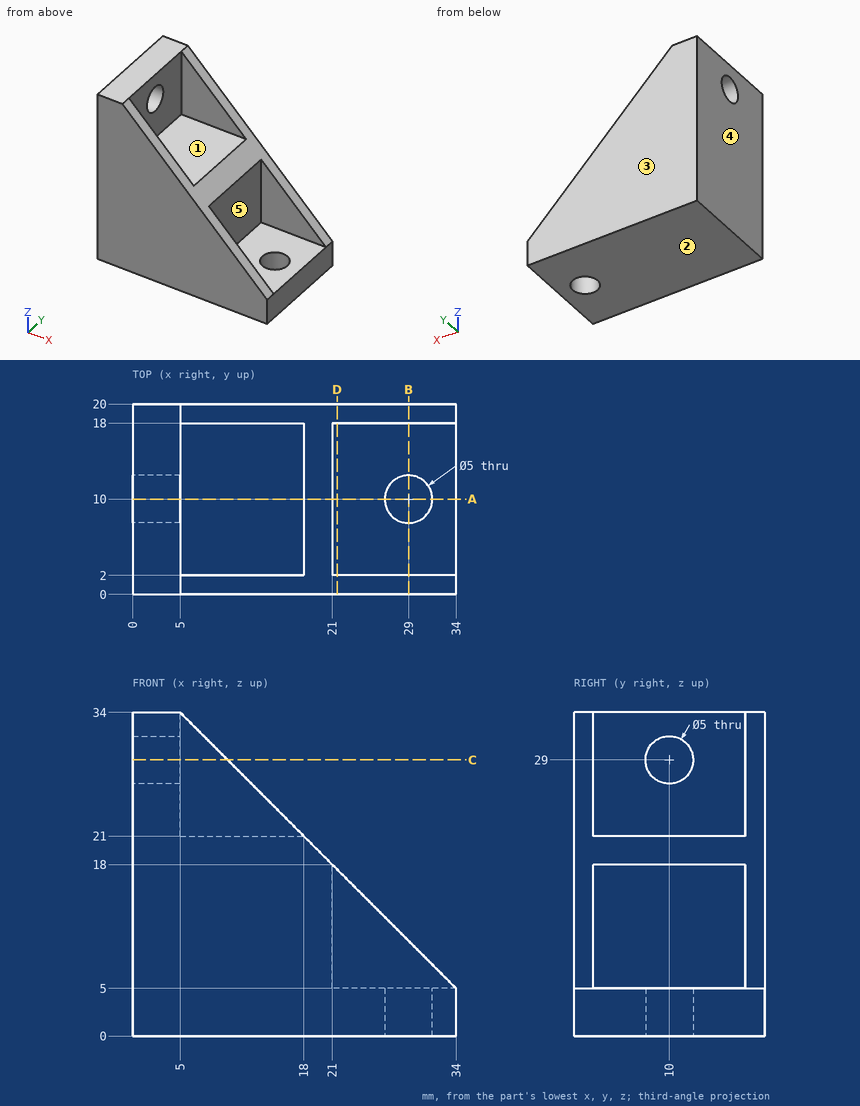
Geometry: see drawing. Coordinates: mm, zero at the bounding-box minimum. A direction names the side the tool comes from. Give positions to 0.01 mm unless a question says otherwise; leave off trailing zeros. Write each loop counter-clockwise with the first axis right and the second up, starting at its lowest first coordinate (ties: lowest second). Pieces come first, ordered by that corner, then holes. Notation, with made-up numbers: (14, 32) - (32, 32) arc R11 ccw to (32, 37) - close; hole circle Ø5 at (66.25, 80.5). An arc over 180 degrees is marked (long way). Return JSON: item names as keys, results as strings. Group by question number.
1) Section C-C on z = 29. Return the cut outline in (x, y).
2) Section B-B on x = 29. Return the cut outline in (y, z).
3) Section A-A on y = 10. Return the cut outline in (x, z), plus the area to 4 significant figures.
4) First-contact query: P1, Ø4, axis at y = 10, z = 10.5, coming from the +X side; P2, Ø10.5, axis at x = 25.5, y = 6, coming from the +Z side; P3, Ø4, axis at x = 9, y = 13, coming from the +Z side. Flat tips, straight axial feed; report the tip coordinate or a pass-through.
5) Line query: line 1 (Y direction, x = 8, z = 24); line 2 (Y direction, x = 29, z = 1); line 3 (Z direction, x = 23, y = 13.5). Output: solid intervals per line, ascending.
6) Section D-D on x = 21.5. Return the cut outline in (y, z).
7) Mould query, pull axis Y, two halves, no side actions, for the marked faces 3, 4 and 5. Classes: released by +Y, released by -Y, zero draft, split by the parting line, or undercut.
8) Set-up query: the marked faces 1 and 2. Return all of +Z, -Z, +X, -X, +Y, -Y with unobstructed straight access to the full face (end or side cutting, diameter ignored); none if empty.
Filled in:
{
 "1": {"outline": "(0, 0) - (10, 0) - (10, 2) - (5, 2) - (5, 7.5) - (0, 7.5) - close; (0, 12.5) - (5, 12.5) - (5, 18) - (10, 18) - (10, 20) - (0, 20) - close"},
 "2": {"outline": "(0, 0) - (7.5, 0) - (7.5, 5) - (2, 5) - (2, 10) - (0, 10) - close; (12.5, 0) - (20, 0) - (20, 10) - (18, 10) - (18, 5) - (12.5, 5) - close"},
 "3": {"outline": "(0, 0) - (26.5, 0) - (26.5, 5) - (21, 5) - (21, 18) - (18, 21) - (5, 21) - (5, 26.5) - (0, 26.5) - close; (0, 31.5) - (5, 31.5) - (5, 34) - (0, 34) - close; (31.5, 0) - (34, 0) - (34, 5) - (31.5, 5) - close", "area": "516.5 mm^2"},
 "4": {"P1": "stops at x = 21", "P2": "stops at z = 18.75", "P3": "stops at z = 21"},
 "5": {"line 1": "y = 0 to 2, 18 to 20", "line 2": "y = 0 to 7.5, 12.5 to 20", "line 3": "z = 0 to 5"},
 "6": {"outline": "(0, 0) - (20, 0) - (20, 17.5) - (18, 17.5) - (18, 5) - (2, 5) - (2, 17.5) - (0, 17.5) - close"},
 "7": {"face 3": "released by +Y", "face 4": "zero draft", "face 5": "undercut"},
 "8": {"face 1": "+Z, +X", "face 2": "-Z, +X, -X, +Y, -Y"}
}
